Geometry: final body of the model. Coordinates: model frame, mm. Face numbers are marked on the shaded views. A direction names the side the tool comes from. Give positions to 0.01 mm unless a question says otherwise; leave off trailing zeros. Write each loop counter-clockwise with the first axis right and the second up, starting at its lowest first coordinate (ties: lowest second). Pieces come first, ordered by that corner, then holes.
```python
from build123d import *

# Parameters (mm, degrees)
F1_DEPTH = 11.95
F2_R     = 2.5
F3_DEPTH = 4.75
F4_W     = 3.5
F4_H     = 22
F5_DEPTH = 12.5
F6_W     = 3
F6_H     = 10
F7_DEPTH = 3
F8_SIZE  = 1


with BuildPart() as f1:
    # F0 (on Front) → F1 (new body, symmetric)
    with BuildSketch(Plane.XZ):
        Polygon((-15.25, 1.65), (-12.25, 1.65), (-12.25, 4.45), (-18.25, 4.45), (-18.25, -3.65), (18.25, -3.65), (18.25, 4.45), (17.25, 4.45), (14.25, 3.15), (14.25, 1.65), (15.25, 1.65), (15.25, -1.65), (-15.25, -1.65), align=None)
    extrude(amount=F1_DEPTH, both=True)

    # F2 (on Front) → F3 (join, symmetric)
    with BuildSketch(Plane.XZ):
        with BuildLine():
            Line((-9, -3.65), (-9, -11.65))
            ThreePointArc((-9, -11.65), (-1.883452, -19.60107), (6.804878, -13.406098))
            Line((6.804878, -13.406098), (9, -3.65))
            Line((9, -3.65), (-9, -3.65))
        make_face()
        with Locations((-1, -11.65)):
            Circle(F2_R, mode=Mode.SUBTRACT)
    extrude(amount=F3_DEPTH, both=True)

    # F4 (on Right) → F5 (cut, symmetric)
    with BuildSketch(Plane.YZ):
        with Locations((0, -14.65)):
            Rectangle(F4_W, F4_H)
    extrude(amount=F5_DEPTH, both=True, mode=Mode.SUBTRACT)

    # F6 (on face) → F7 (join)
    with BuildSketch(Plane(origin=(0, 0, -3.65), x_dir=(1, 0, 0), z_dir=(0, 0, -1))):
        with Locations((19.75, 0)):
            Rectangle(F6_W, F6_H)
        with BuildLine():
            Line((21.25, 5), (21.25, -5))
            ThreePointArc((21.25, -5), (26.25, 0), (21.25, 5))
        make_face()
    extrude(amount=-F7_DEPTH)

    # F8
    f8_edges = [f1.edges().sort_by_distance(p)[0] for p in [
        (26.25, 0, -0.65),
    ]]
    chamfer(f8_edges, length=F8_SIZE)


solid = f1.part
```
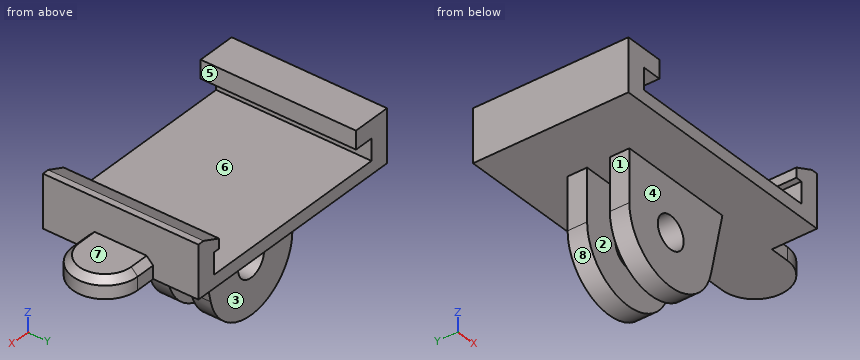
Item 1: Pull-direction query (X, two-part tool) for the marked faces 5, 6, 7 and 8; classes: +X half, -X half, draft (parallel to the pull), parting line (faces both ways), or undercut.
Found:
face 5: undercut
face 6: undercut
face 7: draft
face 8: parting line
Item 2: Pin query (flat end, axial travel): pin 1 Ø1.4 at (y, z) = (-5.5, 3) entering from +X; pin 2 Ø3.5 at (x, y) = (20.5, 1.5) entering from +Z; pin 3 Ø1.5 at (x, y) = (-13.5, -1) entering from -Z. Return the tip coordinate at first contact, or that it passes through.
Found:
pin 1: stops at x = 18.25
pin 2: stops at z = -0.65
pin 3: stops at z = -3.65
Item 3: Section A-A, the plane x = -1. Return the cut outline in (y, z).
Found:
outline: (-11.95, -3.65) - (-4.75, -3.65) - (-4.75, -9.15) - (-1.75, -9.15) - (-1.75, -3.65) - (1.75, -3.65) - (1.75, -9.15) - (4.75, -9.15) - (4.75, -3.65) - (11.95, -3.65) - (11.95, -1.65) - (-11.95, -1.65) - close; (-4.75, -19.65) - (-1.75, -19.65) - (-1.75, -14.15) - (-4.75, -14.15) - close; (1.75, -19.65) - (4.75, -19.65) - (4.75, -14.15) - (1.75, -14.15) - close
Item 4: Section B-B, the plane x = -13. Return the cut outline in (y, z), plus the area to 3 significant figures.
Found:
outline: (-11.95, -3.65) - (11.95, -3.65) - (11.95, -1.65) - (-11.95, -1.65) - close; (-11.95, 1.65) - (11.95, 1.65) - (11.95, 4.45) - (-11.95, 4.45) - close
area: 115 mm2
Item 5: Section C-C, the plane z = -5.5. Return the cut outline in (x, y), plus the area to 3 significant figures.
Found:
outline: (-9, -4.75) - (8.58, -4.75) - (8.58, -1.75) - (-9, -1.75) - close; (-9, 1.75) - (8.58, 1.75) - (8.58, 4.75) - (-9, 4.75) - close
area: 106 mm2
Item 6: Reachability of the marked faces 1, 2, 3 and 4 from +Z, -Z, +X, -X, +Y, -Y: full face, straight path, thin tool, end or side. Return the list, or none.
Found:
face 1: -Z, -X, +Y, -Y
face 2: -Z, +X, -X
face 3: -Z, +X, -X, +Y
face 4: -Z, +X, -X, -Y
Item 7: Section D-D, the plane y = 6.5. Return the cut outline in (x, z), plus the area to 3 significant figures.
Found:
outline: (-18.25, -3.65) - (18.25, -3.65) - (18.25, 4.45) - (17.25, 4.45) - (14.25, 3.15) - (14.25, 1.65) - (15.25, 1.65) - (15.25, -1.65) - (-15.25, -1.65) - (-15.25, 1.65) - (-12.25, 1.65) - (-12.25, 4.45) - (-18.25, 4.45) - close
area: 119 mm2
Item 8: Line query: L1, parallel to X at y = 10.5, z = -0.25; L2, parallel to Z at x = -1, y = -3.25; L3, parallel to X at y = -9.5, z = 1.75. Output: solid intervals per line, ascending.
Found:
L1: x = -18.25 to -15.25, 15.25 to 18.25
L2: z = -19.65 to -14.15, -9.15 to -1.65
L3: x = -18.25 to -12.25, 14.25 to 18.25
